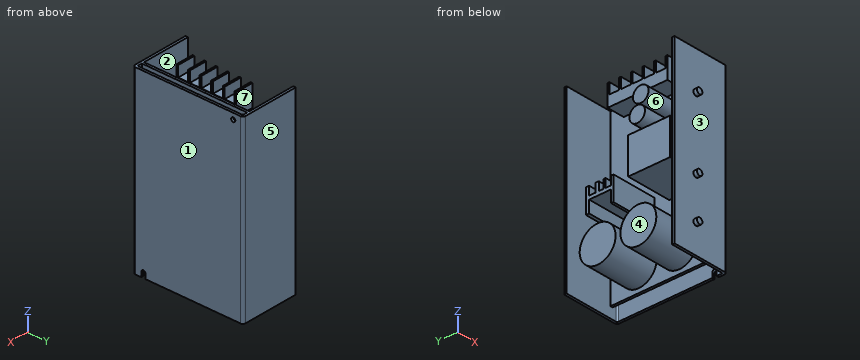
from build123d import *

# Parameters (mm, degrees)
EXTRUDE_1_DEPTH     = 150
SKETCH_2_W          = 2
SKETCH_2_H          = 88
EXTRUDE_2_DEPTH     = 150
SKETCH_3_R          = 15
SKETCH_3_R_2        = 6.5
SKETCH_3_W          = 30
SKETCH_3_H          = 35
EXTRUDE_3_DEPTH     = 38
EXTRUDE_4_DEPTH     = 15
CUT_EXTRUDE_1_REACH = 174.877
SKETCH_5_R          = 1.75
SKETCH_6_R          = 2.5
EXTRUDE_5_DEPTH     = 3
CUT_EXTRUDE_2_REACH = 173.633
SKETCH_7_W          = 9
SKETCH_7_H          = 88


with BuildPart() as part:
    # 草图1 → 凸台-拉伸1 (new body)
    with BuildSketch(Plane.XY):
        with BuildLine():
            Line((-24.3, 44), (21.3, 44))
            ThreePointArc((21.3, 44), (22.007106781, 43.707106781), (22.3, 43))
            Line((22.3, 43), (22.3, -43))
            ThreePointArc((22.3, -43), (22.007106781, -43.707106781), (21.3, -44))
            Line((21.3, -44), (-24.3, -44))
            Line((-24.3, -44), (-24.3, -46))
            Line((-24.3, -46), (22.3, -46))
            ThreePointArc((22.3, -46), (23.714213562, -45.414213562), (24.3, -44))
            Line((24.3, -44), (24.3, 44))
            ThreePointArc((24.3, 44), (23.714213562, 45.414213562), (22.3, 46))
            Line((22.3, 46), (-24.3, 46))
            Line((-24.3, 46), (-24.3, 44))
        make_face()
    extrude(amount=EXTRUDE_1_DEPTH)

    # 草图2 → 凸台-拉伸2 (add)
    with BuildSketch(Plane(origin=(0, 0, 0), x_dir=(-1, 0, 0), z_dir=(0, 0, -1))):
        with Locations((-17.3, 0)):
            Rectangle(SKETCH_2_W, SKETCH_2_H)
    extrude(amount=-EXTRUDE_2_DEPTH)

    # 草图3 → 凸台-拉伸3 (add)
    with BuildSketch(Plane.ZY.offset(-16.3)):
        with Locations(Location((27.5, 20.5, 0), (0, 0, 270))):
            Circle(SKETCH_3_R)
        with Locations(Location((27.5, -13.5, 0), (0, 0, 270))):
            Circle(SKETCH_3_R)
        with Locations(Location((108.160228903, -12.5, 0), (0, 0, 270))):
            Circle(SKETCH_3_R_2)
        with Locations(Location((121.5, -15.5, 0), (0, 0, 270))):
            Circle(SKETCH_3_R_2)
        with Locations((81, -22.5)):
            Rectangle(SKETCH_3_W, SKETCH_3_H)
        Polygon((52.497113206, 30.367528908), (72.528628507, 30.367528908), (72.528628507, 27.598945493), (65.398687695, 27.598945493), (65.398687695, 22.22463651), (72.528628507, 22.22463651), (72.528628507, 19.456053094), (65.398687695, 19.456053094), (65.398687695, 15.547464743), (72.528628507, 15.547464743), (72.528628507, 13.756028415), (65.398687695, 13.756028415), (65.398687695, 9.196008671), (72.528628507, 9.196008671), (72.528628507, 7.241714496), (52.497113206, 7.241714496), (52.497113206, 9.196008671), (62.512870856, 9.196008671), (62.512870856, 27.598945493), (52.497113206, 27.598945493), align=None)
    extrude(amount=EXTRUDE_3_DEPTH)

    # 草图4 → 凸台-拉伸4 (add)
    with BuildSketch(Plane.ZY.offset(-16.3)):
        Polygon((159.4, 33), (141.4, 33), (141.4, -17), (159.4, -17), (159.4, -15.5), (150.4, -15.5), (150.4, -7.3), (159.4, -7.3), (159.4, -5.8), (150.4, -5.8), (150.4, 2.4), (159.4, 2.4), (159.4, 3.9), (150.4, 3.9), (150.4, 12.1), (159.4, 12.1), (159.4, 13.6), (150.4, 13.6), (150.4, 21.8), (159.4, 21.8), (159.4, 23.3), (150.4, 23.3), (150.4, 31.5), (159.4, 31.5), align=None)
    extrude(amount=EXTRUDE_4_DEPTH)

    # 草图5 → 切除-拉伸1 (cut, up to next)
    with BuildSketch(Plane(origin=(24.3, 0, 0), x_dir=(0, 0, -1), z_dir=(1, 0, 0)), mode=Mode.PRIVATE) as cut_extrude_1_sk1:
        with Locations(Location((-145, 37.7, 0), (0, 0, 90))):
            Circle(SKETCH_5_R)
    cut_extrude_1_tool1 = extrude(cut_extrude_1_sk1.sketch, amount=-CUT_EXTRUDE_1_REACH, mode=Mode.PRIVATE) & part.part
    # 草图5 → 切除-拉伸1 (cut, up to next)
    with BuildSketch(Plane(origin=(24.3, 0, 0), x_dir=(0, 0, -1), z_dir=(1, 0, 0)), mode=Mode.PRIVATE) as cut_extrude_1_sk2:
        with BuildLine():
            Line((-4, -35.55), (0, -35.55))
            Line((0, -35.55), (0, -39.05))
            Line((0, -39.05), (-4, -39.05))
            ThreePointArc((-4, -39.05), (-5.75, -37.3), (-4, -35.55))
        make_face()
    cut_extrude_1_tool2 = extrude(cut_extrude_1_sk2.sketch, amount=-CUT_EXTRUDE_1_REACH, mode=Mode.PRIVATE) & part.part
    add(cut_extrude_1_tool1.solids().sort_by_distance((24.3, 37.7, 145))[0], mode=Mode.SUBTRACT)
    add(cut_extrude_1_tool2.solids().sort_by_distance((24.3, -37.3, 2.701417))[0], mode=Mode.SUBTRACT)

    # 草图6 → 凸台-拉伸5 (add)
    with BuildSketch(Plane.XZ.offset(46)):
        with Locations(Location((-4.3, 118, 0), (0, 0, 180))):
            Circle(SKETCH_6_R)
        with Locations(Location((-4.3, 59, 0), (0, 0, 180))):
            Circle(SKETCH_6_R)
        with Locations(Location((-4.3, 24, 0), (0, 0, 180))):
            Circle(SKETCH_6_R)
    extrude(amount=EXTRUDE_5_DEPTH)

    # 草图7 → 切除-拉伸2 (cut, up to next)
    with BuildSketch(Plane.ZY.offset(-16.3), mode=Mode.PRIVATE) as cut_extrude_2_sk1:
        with Locations((4.5, 0)):
            Rectangle(SKETCH_7_W, SKETCH_7_H)
    cut_extrude_2_tool1 = extrude(cut_extrude_2_sk1.sketch, amount=-CUT_EXTRUDE_2_REACH, mode=Mode.PRIVATE) & part.part
    add(cut_extrude_2_tool1.solids().sort_by_distance((16.3, 0, 4.5))[0], mode=Mode.SUBTRACT)


solid = part.part
Model file for the job. Use its own axes, mm. Face numbers are marked on the shaded views. A direction names the side the tool comes from. Give positions to 0.01 mm unless a question says otherwise; leave off trailing zeros. Loops run counter-clockwise (first coordinate to the right, second up) from the corner with the lowest first, then second, coordinate; pieces in that order, holes last.
Item 1: Slice it at C-C (z = 91). Write the cut outline in (x, y), plus the area to 3 significant figures.
Check values:
outline: (-24.3, -46) - (22.3, -46) arc R2 ccw to (24.3, -44) - (24.3, 44) arc R2 ccw to (22.3, 46) - (-24.3, 46) - (-24.3, 44) - (16.3, 44) - (16.3, -5) - (-21.7, -5) - (-21.7, -40) - (16.3, -40) - (16.3, -44) - (-24.3, -44) - close; hole (18.3, -44) - (21.3, -44) arc R1 ccw to (22.3, -43) - (22.3, 43) arc R1 ccw to (21.3, 44) - (18.3, 44) - close
area: 1,880 mm2
Item 2: Mould opens along Y. For the marked faces 1, 2 and 3 say: +Y half, -Y half, draft (parallel to the pull), parting line (faces both ways), or undercut.
Check values:
face 1: draft
face 2: undercut
face 3: -Y half
Item 3: Drop flat-ended pins along their axis: P1, Ø7, axis at x = 7.5, z = 154, coming from the +Y side; P2, Ø1, axis at y = 4, z = 51.5, coming from the -X side; P3, Ø1, axis at x = 23, z = 2, coming from the +Y side. Give the stop position or say it passes through.
Check values:
P1: stops at y = 33
P2: stops at x = 16.3
P3: stops at y = 45.99
Item 4: Slice it at D-D (x = 9). Give the number of separate pieces and of enclosed holes in the cut face, plus the area to 3 significant figures.
Check values:
separate pieces: 9
enclosed holes: 0
area: 4,040 mm2
Item 5: Slice it at A-A (y = -33.5). Write the cut outline in (x, z).
Check values:
outline: (-21.7, 66) - (16.3, 66) - (16.3, 9) - (18.3, 9) - (18.3, 150) - (16.3, 150) - (16.3, 96) - (-21.7, 96) - close; (22.3, 0) - (24.3, 0) - (24.3, 150) - (22.3, 150) - close
Item 6: Slice it at B-B (y = 37.7). Write the cut outline in (x, z).
Check values:
outline: (16.3, 9) - (18.3, 9) - (18.3, 150) - (16.3, 150) - close; (22.3, 0) - (24.3, 0) - (24.3, 143.25) - (22.3, 143.25) - close; (22.3, 146.75) - (24.3, 146.75) - (24.3, 150) - (22.3, 150) - close
Item 7: Which spindle directions (+Z, -Z, +X, -X, +Y, -Y) get a long thin tool onto all of the face, cutting with end or side? Do the marked faces 4, 5, 6 and 7. Say none if no direction does.
Check values:
face 4: +Z, -Z, -X
face 5: +Z, -Z, +X, -X, +Y
face 6: -X
face 7: +Z, -X
Item 8: Drill centre lines: line 1 along Y through (x, z) = (14.5, 87.5); line 2 along Y through (x, z) = (8, 65); line 3 along Y through (x, z) = (14, 59.5). Where is each one in solid material? Low to high.
Check values:
line 1: y = -46 to -44, -40 to -5, 44 to 46
line 2: y = -46 to -44, 7.24 to 30.37, 44 to 46
line 3: y = -46 to -44, 7.24 to 9.2, 27.6 to 30.37, 44 to 46
